Input: part model. Units: mm. Frame: model coordinates. A direction names the side the tool comes from. Give positions to 0.01 mm unless a question says otherwise; leave off trailing zeros. Order: outer loops, then holes, each group sorted by start corner. A loop starts at its lowest first (then second) coordinate and runs counter-clockwise, first axis right, second up. Notation, with made-up numbers: M 67,-30 L 87,-30 A17 ccw 87,-20 Z; hole C 28.25,15.5 d9. An arc over 180 degrees is marked long. Use a Markdown table: item, result.
from build123d import *

# Parameters (mm, degrees)
BOSS_EXTRUDE1_DEPTH = 5
SKETCH2_W           = 3
SKETCH2_H           = 10.5
BOSS_EXTRUDE2_DEPTH = 5
CUT_EXTRUDE1_REACH  = 32.359
SKETCH3_R           = 1.55
SKETCH4_W           = 6.16233047
SKETCH4_H           = 10
SKETCH4_W_2         = 6.16
SKETCH4_W_3         = 17.67766953
BOSS_EXTRUDE3_DEPTH = 5


with BuildPart() as part:
    # Sketch1 → Boss-Extrude1 (new, symmetric)
    with BuildSketch(Plane.XY):
        with BuildLine():
            Line((-15, 15), (-15, 0))
            ThreePointArc((-15, 0), (-10.606601721, 10.606601715), (-8e-09, 15))
            Line((-8e-09, 15), (-15, 15))
        make_face()
        with BuildLine():
            Line((15, 15), (-8e-09, 15))
            ThreePointArc((-8e-09, 15), (10.606601715, 10.606601721), (15, 0))
            Line((15, 0), (15, 15))
        make_face()
        with BuildLine():
            ThreePointArc((-8e-09, 15), (-10.606601721, 10.606601715), (-15, 0))
            ThreePointArc((-15, 0), (-11.039701083, -10.155048006), (-1.25, -14.947825929))
            Line((-1.25, -14.947825929), (-1.25, -12.437342964))
            ThreePointArc((-1.25, -12.437342964), (-8.385254916, 9.270248109), (12.5, 0))
            ThreePointArc((12.5, 0), (9.270248109, -8.385254916), (1.25, -12.437342964))
            Line((1.25, -12.437342964), (1.25, -14.947825929))
            ThreePointArc((1.25, -14.947825929), (11.039701083, -10.155048006), (15, 0))
            ThreePointArc((15, 0), (10.606601715, 10.606601721), (-8e-09, 15))
        make_face()
    extrude(amount=BOSS_EXTRUDE1_DEPTH, both=True)

    # Sketch2 → Boss-Extrude2 (add, symmetric)
    with BuildSketch(Plane.XY):
        with Locations((-2.75, -17.687342964)):
            Rectangle(SKETCH2_W, SKETCH2_H)
        with Locations((2.75, -17.687342964)):
            Rectangle(SKETCH2_W, SKETCH2_H)
    extrude(amount=BOSS_EXTRUDE2_DEPTH, both=True)

    # Cut-Extrude1: up to this face of the body (flat: up to its plane)
    cut_extrude1_end = Plane(part.part.faces().sort_by_distance((4.25, -18.661332672, 0))[0])
    # Sketch3 → Cut-Extrude1 (cut, up to the picked face)
    with BuildSketch(Plane.ZY.offset(4.25), mode=Mode.PRIVATE) as cut_extrude1_sk1:
        with Locations(Location((0, -18.385322381, 0), (0, 0, 270))):
            Circle(SKETCH3_R)
    cut_extrude1_tool1 = split(extrude(cut_extrude1_sk1.sketch, amount=-CUT_EXTRUDE1_REACH, mode=Mode.PRIVATE), bisect_by=cut_extrude1_end, keep=Keep.BOTH, mode=Mode.PRIVATE)
    add(cut_extrude1_tool1.solids().sort_by(Axis((-4.25, -18.385322, 0), (1, 0, 0)))[0], mode=Mode.SUBTRACT)

    # Sketch4 → Boss-Extrude3 (add)
    with BuildSketch(Plane(origin=(0, 15, 0), x_dir=(1, 0, 0), z_dir=(0, 1, 0))):
        with BuildLine():
            Line((15, 15), (-15, 15))
            Line((-15, 15), (-15, 5))
            Line((-15, 5), (-8.84, 5))
            Line((-8.84, 5), (-8.84, 7.34))
            ThreePointArc((-8.84, 7.34), (-9.900660172, 9.900660172), (-7.34, 8.84))
            Line((-7.34, 8.84), (7.33766953, 8.84))
            ThreePointArc((7.33766953, 8.84), (8.83766953, 10.34), (10.33766953, 8.84))
            ThreePointArc((10.33766953, 8.84), (9.898329701, 7.779339828), (8.83766953, 7.34))
            Line((8.83766953, 7.34), (8.83766953, 5))
            Line((8.83766953, 5), (15, 5))
            Line((15, 5), (15, 15))
        make_face()
        with Locations((11.918834765, 0)):
            Rectangle(SKETCH4_W, SKETCH4_H)
        with BuildLine():
            Line((-8.84, -5), (-15, -5))
            Line((-15, -5), (-15, -15))
            Line((-15, -15), (15, -15))
            Line((15, -15), (15, -5))
            Line((15, -5), (8.83766953, -5))
            Line((8.83766953, -5), (8.83766953, -7.33766953))
            ThreePointArc((8.83766953, -7.33766953), (9.898329701, -7.777009358), (10.33766953, -8.83766953))
            ThreePointArc((10.33766953, -8.83766953), (8.83766953, -10.33766953), (7.33766953, -8.83766953))
            Line((7.33766953, -8.83766953), (-7.34, -8.83766953))
            ThreePointArc((-7.34, -8.83766953), (-9.900660172, -9.898329701), (-8.84, -7.33766953))
            Line((-8.84, -7.33766953), (-8.84, -5))
        make_face()
        with Locations((-11.92, 0)):
            Rectangle(SKETCH4_W_2, SKETCH4_H)
        with BuildLine():
            Line((8.83766953, -5), (-8.84, -5))
            Line((-8.84, -5), (-8.84, -7.33766953))
            ThreePointArc((-8.84, -7.33766953), (-7.779339828, -7.777009358), (-7.34, -8.83766953))
            Line((-7.34, -8.83766953), (7.33766953, -8.83766953))
            ThreePointArc((7.33766953, -8.83766953), (7.777009358, -7.777009358), (8.83766953, -7.33766953))
            Line((8.83766953, -7.33766953), (8.83766953, -5))
        make_face()
        with Locations((-0.001165235, 0)):
            Rectangle(SKETCH4_W_3, SKETCH4_H)
        with BuildLine():
            Line((-8.84, 7.34), (-8.84, 5))
            Line((-8.84, 5), (8.83766953, 5))
            Line((8.83766953, 5), (8.83766953, 7.34))
            ThreePointArc((8.83766953, 7.34), (7.777009358, 7.779339828), (7.33766953, 8.84))
            Line((7.33766953, 8.84), (-7.34, 8.84))
            ThreePointArc((-7.34, 8.84), (-7.779339828, 7.779339828), (-8.84, 7.34))
        make_face()
    extrude(amount=BOSS_EXTRUDE3_DEPTH)


solid = part.part
1) Cut plane D-D on x = 0. Return loops of the section in (y, z), and give its area (3 significant figures).
Response values:
| item | result |
|---|---|
| outline | M 12.5,-5 L 15,-5 L 15,-15 L 20,-15 L 20,15 L 15,15 L 15,5 L 12.5,5 Z |
| area | 175 mm² |
2) Material intervals for line 1 (X direction, y = -17.5, z = -4.75); line 2 (Z direction, x = -8.84, y = 17.3); line 3 (X direction, y = 15.5, z = -9), sorted ascending. Write a range as from..to.
Response values:
| item | result |
|---|---|
| line 1 | x = -4.25..-1.25, 1.25..4.25 |
| line 2 | z = -15..-10.34, -7.34..7.34, 10.34..15 |
| line 3 | x = -15..-10.33, -7.35..7.35, 10.33..15 |
3) Cut plane C-C on x = 3. Return loops of the section in (y, z), and give its area (3 significant figures).
Response values:
| item | result |
|---|---|
| outline | M -22.94,-5 L -12.13,-5 L -12.13,5 L -22.94,5 Z; M 12.13,-5 L 15,-5 L 15,-15 L 20,-15 L 20,15 L 15,15 L 15,5 L 12.13,5 Z; hole C -18.39,0 d3.1 |
| area | 279 mm² |
4) First-contact query: pin 1 Ø8 at (x, y) = (-10, -10) entering from -Z; pin 2 Ø2.5 at (y, z) = (-20.5, 0) entering from -X; pin 3 Ø8 at (x, z) = (-5.5, -8.5) entering from -Y; pin 4 Ø9.5 at (y, z) = (-18, -1.5) entering from +X. Flat tips, straight axial feed; report the tip coordinate or a pass-through.
Response values:
| item | result |
|---|---|
| pin 1 | stops at z = -5 |
| pin 2 | stops at x = -4.25 |
| pin 3 | stops at y = -22.94 |
| pin 4 | stops at x = 7.03 |
5) Cut plane A-A on z = 0. Return loops of the section in (x, y), and give its area (3 significant figures).
Response values:
| item | result |
|---|---|
| outline | M -15,0 A15 ccw -4.25,-14.39 L -4.25,-16.84 L -1.25,-16.84 L -1.25,-12.44 A12.5 cw long 1.25,-12.44 L 1.25,-16.84 L 4.25,-16.84 L 4.25,-14.39 A15 ccw 15,0 L 15,20 L -15,20 Z; M -4.25,-22.94 L -1.25,-22.94 L -1.25,-19.94 L -4.25,-19.94 Z; M 1.25,-22.94 L 4.25,-22.94 L 4.25,-19.94 L 1.25,-19.94 Z |
| area | 487 mm² |
6) Cut plane B-B on y = 0.5. Return loops of the section in (x, z), and give its area (3 significant figures).
Response values:
| item | result |
|---|---|
| outline | M -15,-5 L -12.49,-5 L -12.49,5 L -15,5 Z; M 12.49,-5 L 15,-5 L 15,5 L 12.49,5 Z |
| area | 50.2 mm² |
7) Reachability of faces 5 (the face through (-9, 9, -5)), 6 (the face through (4.25, -20, -1)), 7 (the face through (0, 15, 10)), 8 (the face through (-4.25, -20, 1)), 9 (the face through (-2.771, -16.837, 0.068)) from +Z, -Z, +X, -X, +Y, -Y: full face, straight path, thin tool, end or side. Return the list, or none.
Response values:
| item | result |
|---|---|
| face 5 | -Z, +X, -X, -Y |
| face 6 | +Z, -Z, +X, -Y |
| face 7 | +Z, +X, -X, -Y |
| face 8 | +Z, -Z, -X, -Y |
| face 9 | +X, -X |
8) Mould query, pull axis X, two halves, no side actions, for faces 1 (the face through (15, 12, 0)), 2 (the face through (-3, -22.937, 0)), 3 (the face through (1.25, -16.6, 0.1)), 4 (the face through (-1.25, -16.6, 0.1)). Classes: released by +X, released by -X, zero draft, split by the parting line, or undercut.
Response values:
| item | result |
|---|---|
| face 1 | released by +X |
| face 2 | zero draft |
| face 3 | undercut |
| face 4 | undercut |
